from build123d import *

# Parameters (mm, degrees)
SKETCH3_R          = 1.5
CUT_EXTRUDE1_DEPTH = 89.36854644


with BuildPart() as part:
    # Sketch2 → Revolve1 (revolve)
    with BuildSketch(Plane.XY):
        Polygon((0, 5), (0, 0), (50, 0), (50, 5), (41, 5), (41, 58), (38, 58), (38, 5), align=None)
    revolve(axis=Axis((0, 0, 0), (0, 1, 0)))

    # Sketch3 → Cut-Extrude1 (cut, through all)
    with BuildSketch(Plane(origin=(0, 5, 0), x_dir=(1, 0, 0), z_dir=(0, 1, 0))):
        with Locations(Location((-13.5, 4, 0), (0, 0, 180))):
            Circle(SKETCH3_R)
        with Locations(Location((13.5, 4, 0), (0, 0, 180))):
            Circle(SKETCH3_R)
        with Locations(Location((-13.5, -4, 0), (0, 0, 180))):
            Circle(SKETCH3_R)
        with Locations(Location((-13.5, -12, 0), (0, 0, 180))):
            Circle(SKETCH3_R)
        with Locations(Location((13.5, -4, 0), (0, 0, 180))):
            Circle(SKETCH3_R)
        with Locations(Location((13.5, -12, 0), (0, 0, 180))):
            Circle(SKETCH3_R)
        with Locations(Location((-13.5, 12, 0), (0, 0, 180))):
            Circle(SKETCH3_R)
        with Locations(Location((13.5, 12, 0), (0, 0, 180))):
            Circle(SKETCH3_R)
        with Locations(Location((0, -47, 0), (0, 0, 180))):
            Circle(SKETCH3_R)
        with Locations(Location((-33.234018716, -33.234018716, 0), (0, 0, 180))):
            Circle(SKETCH3_R)
        with Locations(Location((-47, 0, 0), (0, 0, 180))):
            Circle(SKETCH3_R)
        with Locations(Location((-33.234018716, 33.234018716, 0), (0, 0, 180))):
            Circle(SKETCH3_R)
        with Locations(Location((0, 47, 0), (0, 0, 180))):
            Circle(SKETCH3_R)
        with Locations(Location((33.234018716, 33.234018716, 0), (0, 0, 180))):
            Circle(SKETCH3_R)
        with Locations(Location((47, 0, 0), (0, 0, 180))):
            Circle(SKETCH3_R)
        with Locations(Location((33.234018716, -33.234018716, 0), (0, 0, 180))):
            Circle(SKETCH3_R)
    extrude(amount=-CUT_EXTRUDE1_DEPTH, mode=Mode.SUBTRACT)


solid = part.part
Part model, mm, in its own coordinate system. A direction names the side the tool comes from. Coordinates: 2 decimals unless noted, no trailing zeros. Loops run counter-clockwise (first coordinate to the right, second up) from the corner with the lowest first, then second, coordinate; pieces in that order, holes last. Notation, with made-up numbers: M 70.5,14.5 L 85.5,14.5 A19 cw 85.5,51.5 Z; hole C 69.5,-32.5 d3. An arc over 180 degrees is marked long. Use a Markdown table: item, result. Add a question column.
Q1. Cut at C-C (z = -47). Write the cut outline in (x, y).
Q2. Cut at A-A (z = 0). Write the cut outline in (x, y), and give its area (3 significant figures).
Q3. Which spindle directions (+Z, -Z, +X, -X, +Y, -Y) get a long thin tool onto all of the face, cutting with end or side? Do faces 4 (the cylindrical face through (17.535, 31.129, 33.713)), 5 (the cylindrical face through (-12, 3, -12)). Say none if no direction does.
Q4. Cut at B-B (x = 47). Write the cut outline in (y, z), and give its area (3 significant figures).
Q5. Cut at D-D (x = 13.5). Write the cut outline in (y, z), and give its area (3 significant figures).
Q6. Mould opens along Z. For faces 1 (the cylindrical face through (-33.039, 2.535, -31.747)), 2 (the cylindrical face through (-9, 32, 40)), 3 (the flat face through (12, 58, 36.3)) say: +Z half, -Z half, draft (parallel to the pull), parting line (faces both ways), or undercut.
Q7. Probe L1, parallel to Z at x = -13, y = 1; L2, parallel to Z at x = 0, y = 1.6; L3, parallel to Z at x = -1, y = 7. List the from-to ranges inside material, lowest first.
Q8. Pin check, flat tips, straight feed: P1, Ø8, axis at y = 15.5, z = 34.5, coming from the -X side; P2, Ø4, axis at x = 0, z = 47, coming from the -Y side; P3, Ø1, axis at x = 34.5, z = 4, coming from the +Y side; P4, Ø5, axis at x = -1, y = 50, coming from the +Z side. Stop position of each tip, or through.
Worked out:
| question | item | result |
|---|---|---|
| 1 | outline | M -17.06,0 L -1.5,0 L -1.5,5 L -17.06,5 Z; M 1.5,0 L 17.06,0 L 17.06,5 L 1.5,5 Z |
| 2 | outline | M -50,0 L -48.5,0 L -48.5,5 L -50,5 Z; M -45.5,0 L 45.5,0 L 45.5,5 L 41,5 L 41,58 L 38,58 L 38,5 L -38,5 L -38,58 L -41,58 L -41,5 L -45.5,5 Z; M 48.5,0 L 50,0 L 50,5 L 48.5,5 Z |
| 2 | area | 788 mm2 |
| 3 | face 4 | +Y |
| 3 | face 5 | +Y, -Y |
| 4 | outline | M 0,-17.06 L 5,-17.06 L 5,-1.5 L 0,-1.5 Z; M 0,1.5 L 5,1.5 L 5,17.06 L 0,17.06 Z |
| 4 | area | 156 mm2 |
| 5 | outline | M 0,-48.14 L 5,-48.14 L 5,-38.71 L 58,-38.71 L 58,-35.52 L 5,-35.52 L 5,-13.5 L 0,-13.5 Z; M 0,-10.5 L 5,-10.5 L 5,-5.5 L 0,-5.5 Z; M 0,-2.5 L 5,-2.5 L 5,2.5 L 0,2.5 Z; M 0,5.5 L 5,5.5 L 5,10.5 L 0,10.5 Z; M 0,13.5 L 5,13.5 L 5,35.52 L 58,35.52 L 58,38.71 L 5,38.71 L 5,48.14 L 0,48.14 Z |
| 5 | area | 760 mm2 |
| 6 | face 1 | undercut |
| 6 | face 2 | parting line |
| 6 | face 3 | draft |
| 7 | L1 | z = -48.28 to -13.41, -10.59 to -5.41, -2.59 to 2.59, 5.41 to 10.59, 13.41 to 48.28 |
| 7 | L2 | z = -50 to -48.5, -45.5 to 45.5, 48.5 to 50 |
| 7 | L3 | z = -40.99 to -37.99, 37.99 to 40.99 |
| 8 | P1 | stops at x = -27.4 |
| 8 | P2 | stops at y = 0 |
| 8 | P3 | stops at y = 5 |
| 8 | P4 | stops at z = 41 |
